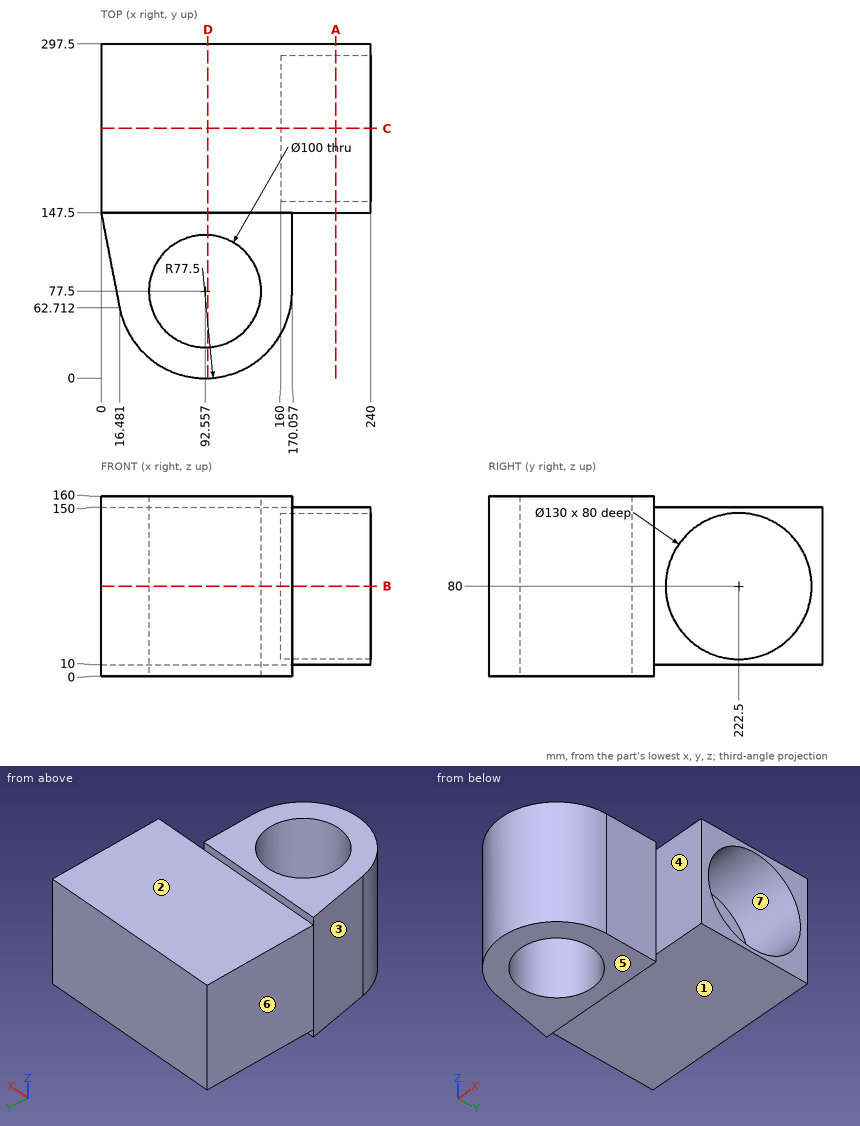
Can you work these out from the drawing? Everything is in mm from the part's minimum corner. A direction names the side the tool comes from. Coordinates: 2 decimals unless noted, no trailing zeros. Write each loop counter-clockwise with the first axis right and the second up, starting at its lowest first coordinate (ties: lowest second). Pieces come first, ordered by that corner, then holes. Notation, with made-up numbers: (54, -13) -> (104, -13) arc R15 cw to (104, 4) -> close; hole circle Ø4 at (-38.75, -22.75). An arc over 180 degrees is marked (long way). Return JSON: item names as keys, results as strings.
(1) Imagine slicing it at A-A, the plane x = 209. Please give me the cut outline in (y, z).
Numbers:
{"outline": "(147.5, 10) -> (297.5, 10) -> (297.5, 150) -> (147.5, 150) -> close; hole circle Ø130 at (222.5, 80)"}
(2) I'm going to push flat-ended pins straight in: pin 1 (8 mm diameter, centred on y = 263, z = 98, fed in from +X); pin 2 (6 mm diameter, centred on x = 199.5, z = 89, fed in from -Y); pin 3 (5 mm diameter, centred on x = 96.5, z = 142, fed in from -Y). Where does each tip first touch, or does it pass through?
Numbers:
{"pin 1": "stops at x = 160", "pin 2": "stops at y = 147.5", "pin 3": "stops at y = 0.01"}
(3) We'd pull the mould along Z, two halves only. Please class the marked faces 5, 6 and 7: +Z half, -Z half, draft (parallel to the pull), parting line (faces both ways), or undercut.
Numbers:
{"face 5": "-Z half", "face 6": "draft", "face 7": "undercut"}
(4) Imagine slicing it at C-C, the plane y = 222.5. Please give me the cut outline in (x, z), then the cut area to 3 significant figures.
Numbers:
{"outline": "(0, 10) -> (240, 10) -> (240, 15) -> (160, 15) -> (160, 145) -> (240, 145) -> (240, 150) -> (0, 150) -> close", "area": "23,200 mm2"}
(5) Imagine slicing it at B-B, the plane z = 80. Please give me the cut outline in (x, y).
Numbers:
{"outline": "(0, 147.5) -> (16.48, 62.71) arc R77.5 ccw to (170.06, 77.5) -> (170.06, 147.5) -> (240, 147.5) -> (240, 157.5) -> (160, 157.5) -> (160, 287.5) -> (240, 287.5) -> (240, 297.5) -> (0, 297.5) -> close; hole circle Ø100 at (92.56, 77.5)"}
(6) Which directions (+Z, -Z, +X, -X, +Y, -Y) give clear straight access to the entire face, cutting with the end or side of a thin tool? Please do the marked faces 1, 2, 3 and 4.
Numbers:
{"face 1": "-Z, +X, -X, +Y", "face 2": "+Z, +X, -X, +Y", "face 3": "+Z, -Z, -X, -Y", "face 4": "+Z, -Z, +X, -Y"}
(7) I need wall thicknesses on L1, parallel to Z at x = 194, y = 222; L2, parallel to Y at x = 199, z = 80; L3, parallel to X at y = 177.5, z = 54. Which ranges of each line are inside material? Lowest first, please.
Numbers:
{"L1": "z = 10 to 15, 145 to 150", "L2": "y = 147.5 to 157.5, 287.5 to 297.5", "L3": "x = 0 to 160"}
(8) Imagine slicing it at D-D, the plane x = 95. Please give me the cut outline in (y, z), then the cut area to 3 significant figures.
Numbers:
{"outline": "(0.04, 0) -> (27.56, 0) -> (27.56, 160) -> (0.04, 160) -> close; (127.44, 0) -> (147.5, 0) -> (147.5, 10) -> (297.5, 10) -> (297.5, 150) -> (147.5, 150) -> (147.5, 160) -> (127.44, 160) -> close", "area": "28,600 mm2"}
